Part model, mm, in its own coordinate system. A direction names the side the tool comes from. Coordinates: 2 decimals unless noted, no trailing zeros. Order: outer loops, then holes, each group sorted by start corner. A loop starts at its lowest first (then second) coordinate and runs counter-clockwise, first axis right, second up.
from build123d import *

# Parameters (mm, degrees)
SKETCH1_W           = 39.5
SKETCH1_H           = 12
SKETCH1_R           = 3.95
BOSS_EXTRUDE1_DEPTH = 4
BOSS_EXTRUDE3_DEPTH = 12
SKETCH4_R           = 1.6
CUT_EXTRUDE1_DEPTH  = 45.55333882
FILLET1_R           = 6
BOSS_EXTRUDE5_DEPTH = 6
SKETCH5_R           = 1.46
BOSS_EXTRUDE4_DEPTH = 4
SKETCH6_W           = 8
SKETCH6_H           = 1
CUT_EXTRUDE3_DEPTH  = 47.786750261


with BuildPart() as part:
    # Sketch1 → Boss-Extrude1 (new body)
    with BuildSketch(Plane.XY):
        with Locations((-3.25, 0)):
            Rectangle(SKETCH1_W, SKETCH1_H)
        Circle(SKETCH1_R, mode=Mode.SUBTRACT)
    extrude(amount=BOSS_EXTRUDE1_DEPTH)

    # Sketch3 → Boss-Extrude3 (add)
    with BuildSketch(Plane.XZ.offset(6)):
        Polygon((-23, 4), (-33, -6), (-43, -6), (-43, -10), (-31.343145751, -10), (-21.343145751, 0), align=None)
    extrude(amount=-BOSS_EXTRUDE3_DEPTH)

    # Sketch4 → Cut-Extrude1 (cut, through all)
    with BuildSketch(Plane.XY.offset(-6)):
        with Locations((-37, 3)):
            Circle(SKETCH4_R)
        with Locations((-37, -3)):
            Circle(SKETCH4_R)
    extrude(amount=-CUT_EXTRUDE1_DEPTH, mode=Mode.SUBTRACT)

    # Fillet1
    fillet1_edges = [part.edges().sort_by_distance(p)[0] for p in [
        (16.5, 6, 2),
        (16.5, -6, 2),
    ]]
    fillet(fillet1_edges, radius=FILLET1_R - 0.0001)  # a hair under: the kernel refuses the full size

    # Sketch7 → Boss-Extrude5 (add)
    with BuildSketch(Plane.XY.offset(4)):
        with BuildLine():
            Line((5.291502622, -6), (10.5, -6))
            ThreePointArc((10.5, -6), (16.5, 0), (10.5, 6))
            Line((10.5, 6), (5.291502622, 6))
            ThreePointArc((5.291502622, 6), (8, 0), (5.291502622, -6))
        make_face()
    extrude(amount=BOSS_EXTRUDE5_DEPTH)

    # Sketch5 → Boss-Extrude4 (add)
    with BuildSketch(Plane.XY.offset(10)):
        with Locations(Location((12.683177793, -3.892819016, 0), (0, 0, 180))):
            Circle(SKETCH5_R)
    extrude(amount=BOSS_EXTRUDE4_DEPTH)

    # Sketch6 → Cut-Extrude3 (cut, through all)
    with BuildSketch(Plane.XZ.offset(6)):
        with Locations((12.5, 0.5)):
            Rectangle(SKETCH6_W, SKETCH6_H)
    extrude(amount=-CUT_EXTRUDE3_DEPTH, mode=Mode.SUBTRACT)


solid = part.part
Q1. Cut at B-B on y = -3. Count the separate pieces of the cut face and the enclosed holes in it, and give its area (3 significant figures).
Results list:
separate pieces: 3
enclosed holes: 0
area: 270 mm2
Q2. Wall check: line 1 along Y through (x, z) = (-37, -7.6); line 2 along Y through (x, z) = (0, 3); line 3 along Z through (x, y) = (-17, -2.75). Give the ranges that are in metal, low to high.
Results list:
line 1: y = -6 to -4.6, -1.4 to 1.4, 4.6 to 6
line 2: y = -6 to -3.95, 3.95 to 6
line 3: z = 0 to 4
Q3. Cut at D-D on z = -7.25. Write the cut outline in (x, y), and give its area (3 significant figures).
Results list:
outline: (-43, -6) - (-28.59, -6) - (-28.59, 6) - (-43, 6) - close; hole circle Ø3.2 at (-37, -3); hole circle Ø3.2 at (-37, 3)
area: 157 mm2
Q4. Which spindle directions (+Z, -Z, +X, -X, +Y, -Y) get a long thin tool onto all of the face, cutting with end or side? Do faces 4 (the face through (8.5, -0.1, 0.5)), 5 (the face through (-28, 0, -1)), 6 (the face through (8, 0, 7)). Say none if no direction does.
Results list:
face 4: -Z, +X, +Y, -Y
face 5: +Z, -X, +Y, -Y
face 6: +Z, -X
Q5. Mould opens along X. For faces 1 (the face through (-38, 0, -6)), 2 (the face through (11.335, -3.334, 11.972)), 3 (the face through (-36.26, 1.58, -7.97)) say: pulls with the +X half, pulls with the -X half, needs draft (parallel to the pull), parting line crosses it, or undercut.
Results list:
face 1: needs draft
face 2: parting line crosses it
face 3: undercut
Q6. Cut at A-A on x = 0. Write the cut outline in (y, z).
Results list:
outline: (-6, 0) - (-3.95, 0) - (-3.95, 4) - (-6, 4) - close; (3.95, 0) - (6, 0) - (6, 4) - (3.95, 4) - close
Q7. Cut at C-C on x = -38. Write the cut outline in (y, z).
Results list:
outline: (-6, -10) - (-4.25, -10) - (-4.25, -6) - (-6, -6) - close; (-1.75, -10) - (1.75, -10) - (1.75, -6) - (-1.75, -6) - close; (4.25, -10) - (6, -10) - (6, -6) - (4.25, -6) - close
Q8. Pin check, flat tips, straight feed: pin 1 Ø5 at (y, z) = (4.5, -6.5) entering from +X; pin 2 Ø8 at (x, z) = (-7, 8.5) entering from +Y; pin 3 Ø6 at (x, y) = (-15, 1) entering from +Z; pin 4 Ø1 at (y, z) = (3, 6) entering from -X. Stop position of each tip, or through.
Results list:
pin 1: stops at x = -25.34
pin 2: passes through
pin 3: stops at z = 4
pin 4: stops at x = 7.19
